```python
from build123d import *

# Parameters (mm, degrees)
ESQUISSE1_W             = 400
ESQUISSE1_H             = 222
BOSS_EXTRU_1_DEPTH      = 340
ESQUISSE2_W             = 356
ESQUISSE2_H             = 318
ENL_V_MAT_EXTRU_1_DEPTH = 462.790308903
ESQUISSE8_W             = 318
ESQUISSE8_H             = 156
ENL_V_MAT_EXTRU_2_DEPTH = 541.935999009
ESQUISSE9_W             = 356
ESQUISSE9_H             = 178
ENL_V_MAT_EXTRU_3_DEPTH = 426.41514362


with BuildPart() as part:
    # Esquisse1 → Boss.-Extru.1 (new body)
    with BuildSketch(Plane.XY):
        with Locations((19.923371648, -19.429118774)):
            Rectangle(ESQUISSE1_W, ESQUISSE1_H)
    extrude(amount=BOSS_EXTRU_1_DEPTH)

    # Esquisse2 → Enlèv. mat.-Extru.1 (cut, through all)
    with BuildSketch(Plane.XZ.offset(130.429118774)):
        with Locations((19.923371648, 159)):
            Rectangle(ESQUISSE2_W, ESQUISSE2_H)
    extrude(amount=-ENL_V_MAT_EXTRU_1_DEPTH, mode=Mode.SUBTRACT)

    # Esquisse8 → Enlèv. mat.-Extru.2 (cut, through all)
    with BuildSketch(Plane(origin=(219.923371648, 0, 0), x_dir=(0, 0, -1), z_dir=(1, 0, 0))):
        with Locations((-159, -8.429118774)):
            Rectangle(ESQUISSE8_W, ESQUISSE8_H)
    extrude(amount=-ENL_V_MAT_EXTRU_2_DEPTH, mode=Mode.SUBTRACT)

    # Esquisse9 → Enlèv. mat.-Extru.3 (cut, through all)
    with BuildSketch(Plane.XY.offset(340)):
        with Locations((19.923371648, -19.429118774)):
            Rectangle(ESQUISSE9_W, ESQUISSE9_H)
    extrude(amount=-ENL_V_MAT_EXTRU_3_DEPTH, mode=Mode.SUBTRACT)


solid = part.part
```
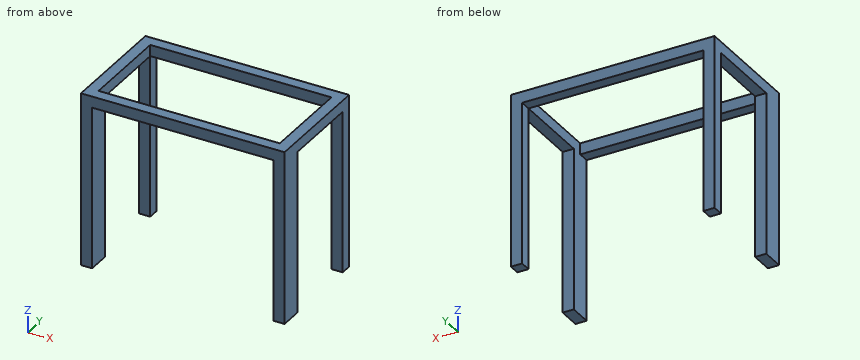
Geometry check sheet. Reference: the model listing, model coordinates, mm. Coordinates: 2 decimals unless noted, no trailing zeros. Loops run counter-clockwise (first coordinate to the right, second up) from the corner with the lowest first, then second, coordinate; pieces in that order, holes last. Notation, with made-up numbers: (72, -6) - (86, -6) arc R29 ccw to (86, 32) - close; hole circle Ø5 at (38, 22). An arc over 180 degrees is marked (long way). One line per item, written item: value. Start each with the question number.
(1) Cross-section at C-C on z = 25.5. Enter the section's corners in (x, y), plus the area to 3 significant figures.
(2) Depth check by flat-ended pin: P1, Ø11, axis at x = -168.5, y = -37.5, coming from the -Z side. Enter the tip coordinate at first touch or a pass-through.
(3) Cross-section at B-B on x = -149.5. Enter the section's corners in (y, z).
(4) Material ranges on line 1 (Z direction, x = -123.5, y = 78), recorded low to high. Write a range as [from, to].
(5) Cross-section at A-A on y = 19. Enter the section's corners in (x, z).
Results below:
1. outline: (-180.08, -130.43) - (-158.08, -130.43) - (-158.08, -86.43) - (-180.08, -86.43) - close; (-180.08, 69.57) - (-158.08, 69.57) - (-158.08, 91.57) - (-180.08, 91.57) - close; (197.92, -130.43) - (219.92, -130.43) - (219.92, -86.43) - (197.92, -86.43) - close; (197.92, 69.57) - (219.92, 69.57) - (219.92, 91.57) - (197.92, 91.57) - close
1. area: 2,900 mm2
2. P1: stops at z = 318
3. outline: (-130.43, 318) - (-108.43, 318) - (-108.43, 340) - (-130.43, 340) - close; (69.57, 318) - (91.57, 318) - (91.57, 340) - (69.57, 340) - close
4. line 1: z = [318, 340]
5. outline: (-180.08, 318) - (-158.08, 318) - (-158.08, 340) - (-180.08, 340) - close; (197.92, 318) - (219.92, 318) - (219.92, 340) - (197.92, 340) - close
